```python
from build123d import *

# Parameters (mm, degrees)
EXTRUDE_1_DEPTH     = 10
EXTRUDE_2_DEPTH     = 13
EXTRUDE_3_DEPTH     = 9
EXTRUDE_4_DEPTH     = 9
SKETCH_7_R          = 74.5
SKETCH_7_R_2        = 62
EXTRUDE_5_DEPTH     = 16
SKETCH_8_R          = 62
CUT_EXTRUDE_1_DEPTH = 10
SKETCH_9_R          = 15
CUT_EXTRUDE_2_DEPTH = 10
SKETCH_10_R         = 2.5
CUT_EXTRUDE_3_DEPTH = 10
SKETCH_11_R         = 2.1
CUT_EXTRUDE_4_DEPTH = 10
SKETCH_12_R         = 2.5
CUT_EXTRUDE_5_DEPTH = 16
SKETCH_14_R         = 7
CUT_EXTRUDE_7_DEPTH = 13
SKETCH_16_R         = 5
CUT_EXTRUDE_9_DEPTH = 13


with BuildPart() as part:
    # ｽｹｯﾁ1 → ﾎﾞｽ - 押し出し1 (new body)
    with BuildSketch(Plane.XY):
        with BuildLine():
            Line((13, 0), (308, 0))
            Line((308, 0), (318, 10))
            Line((318, 10), (318, 348))
            Line((318, 348), (308, 358))
            Line((308, 358), (13, 358))
            Line((13, 358), (13, 214))
            Line((13, 214), (56, 214))
            ThreePointArc((56, 214), (63.071067812, 211.071067812), (66, 204))
            Line((66, 204), (66, 154))
            ThreePointArc((66, 154), (63.071067812, 146.928932188), (56, 144))
            Line((56, 144), (13, 144))
            Line((13, 144), (13, 0))
        make_face()
    extrude(amount=-EXTRUDE_1_DEPTH)

    # ｽｹｯﾁ2 → ﾎﾞｽ - 押し出し2 (add)
    with BuildSketch(Plane(origin=(0, 0, 0), x_dir=(0, 0, -1), z_dir=(1, 0, 0))):
        with BuildLine():
            Line((0, 0), (108, 0))
            ThreePointArc((108, 0), (115.071067812, 2.928932188), (118, 10))
            Line((118, 10), (118, 348))
            ThreePointArc((118, 348), (115.071067812, 355.071067812), (108, 358))
            Line((108, 358), (0, 358))
            Line((0, 358), (0, 0))
        make_face()
    extrude(amount=EXTRUDE_2_DEPTH)

    # ｽｹｯﾁ4 → ﾎﾞｽ - 押し出し3 (add)
    with BuildSketch(Plane(origin=(0, 40, 0), x_dir=(1, 0, 0), z_dir=(0, 1, 0))):
        Polygon((13, 10), (318, 10), (318, 108), (308, 118), (13, 118), align=None)
    extrude(amount=EXTRUDE_3_DEPTH)

    # ｽｹｯﾁ6 → ﾎﾞｽ - 押し出し4 (add)
    with BuildSketch(Plane(origin=(0, 309, 0), x_dir=(1, 0, 0), z_dir=(0, 1, 0))):
        Polygon((13, 10), (318, 10), (318, 108), (308, 118), (13, 118), align=None)
    extrude(amount=EXTRUDE_4_DEPTH)

    # ｽｹｯﾁ7 → ﾎﾞｽ - 押し出し5 (add)
    with BuildSketch(Plane.XY):
        with Locations((228, 179)):
            Circle(SKETCH_7_R)
        with Locations((228, 179)):
            Circle(SKETCH_7_R_2, mode=Mode.SUBTRACT)
    extrude(amount=-EXTRUDE_5_DEPTH)

    # ｽｹｯﾁ8 → ｶｯﾄ - 押し出し1 (cut)
    with BuildSketch(Plane.XY):
        with Locations((228, 179)):
            Circle(SKETCH_8_R)
    extrude(amount=-CUT_EXTRUDE_1_DEPTH, mode=Mode.SUBTRACT)

    # ｽｹｯﾁ9 → ｶｯﾄ - 押し出し2 (cut)
    with BuildSketch(Plane.XY):
        with Locations((122.891, 259.0915)):
            Circle(SKETCH_9_R)
    extrude(amount=-CUT_EXTRUDE_2_DEPTH, mode=Mode.SUBTRACT)

    # ｽｹｯﾁ10 → ｶｯﾄ - 押し出し3 (cut)
    with BuildSketch(Plane.XY):
        with Locations((103.6074, 236.1102)):
            Circle(SKETCH_10_R)
        with Locations((142.1746, 282.0728)):
            Circle(SKETCH_10_R)
    extrude(amount=-CUT_EXTRUDE_3_DEPTH, mode=Mode.SUBTRACT)

    # ｽｹｯﾁ11 → ｶｯﾄ - 押し出し4 (cut)
    with BuildSketch(Plane.XY):
        with Locations((108.5, 14.5)):
            Circle(SKETCH_11_R)
        with Locations((130, 35.5)):
            Circle(SKETCH_11_R)
    extrude(amount=-CUT_EXTRUDE_4_DEPTH, mode=Mode.SUBTRACT)

    # ｽｹｯﾁ12 → ｶｯﾄ - 押し出し5 (cut)
    with BuildSketch(Plane.XY):
        with Locations((295.5, 179)):
            Circle(SKETCH_12_R)
        with Locations((275.7297, 226.7297)):
            Circle(SKETCH_12_R)
        with Locations((228, 246.5)):
            Circle(SKETCH_12_R)
        with Locations((180.2703, 226.7297)):
            Circle(SKETCH_12_R)
        with Locations((160.5, 179)):
            Circle(SKETCH_12_R)
        with Locations((180.2703, 131.2703)):
            Circle(SKETCH_12_R)
        with Locations((228, 111.5)):
            Circle(SKETCH_12_R)
        with Locations((275.7297, 131.2703)):
            Circle(SKETCH_12_R)
    extrude(amount=-CUT_EXTRUDE_5_DEPTH, mode=Mode.SUBTRACT)

    # ｽｹｯﾁ14 → ｶｯﾄ - 押し出し7 (cut)
    with BuildSketch(Plane(origin=(0, 0, 0), x_dir=(0, 0, -1), z_dir=(1, 0, 0))):
        with Locations((30, 15)):
            Circle(SKETCH_14_R)
        with Locations((100, 15)):
            Circle(SKETCH_14_R)
        with Locations((30, 343)):
            Circle(SKETCH_14_R)
        with Locations((100, 343)):
            Circle(SKETCH_14_R)
        with Locations((100, 123)):
            Circle(SKETCH_14_R)
        with Locations((100, 235)):
            Circle(SKETCH_14_R)
    extrude(amount=CUT_EXTRUDE_7_DEPTH, mode=Mode.SUBTRACT)

    # ｽｹｯﾁ16 → ｶｯﾄ - 押し出し9 (cut)
    with BuildSketch(Plane(origin=(0, 0, 0), x_dir=(0, 0, -1), z_dir=(1, 0, 0))):
        with Locations((65, 15)):
            Circle(SKETCH_16_R)
        with Locations((65, 343)):
            Circle(SKETCH_16_R)
    extrude(amount=CUT_EXTRUDE_9_DEPTH, mode=Mode.SUBTRACT)


solid = part.part
```
Design review of the part built by this model. Coordinates are the model's own, in mm. A direction names the side the tool comes from. Round coordinates to 2 decimals unless told otherwise and drop trailing zeros. Write each loop counter-clockwise with the first axis right and the second up, starting at its lowest first coordinate (ties: lowest second). Pieces come first, ordered by that corner, then holes. Notation, with made-up numbers: (74, -9) -> (91, -9) arc R11 cw to (91, 7) -> close; hole circle Ø6 at (54.25, -1). An arc over 180 degrees is marked (long way). Answer in a Markdown table with one row per item.
Q1. Draft analysis for pull direction Y (two halves, no side actions). For faces 4 (the face through (163, 40, -65)), 5 (the face through (163, 318, -65)), 6 (the face through (163, 20, -10)), 7 (the face through (6.41, 10.12, -63.92)), state which applies: +Y half, -Y half, draft (parallel to the pull), parting line (faces both ways), or undercut.
The answers:
| item | result |
|---|---|
| face 4 | -Y half |
| face 5 | +Y half |
| face 6 | draft |
| face 7 | undercut |
Q2. Take a section at B-B, the plane y = 269.5. State the section outline as (x, z) points, then the cut area to 3 significant figures.
The answers:
| item | result |
|---|---|
| outline | (0, -118) -> (13, -118) -> (13, -10) -> (112.09, -10) -> (112.09, 0) -> (0, 0) -> close; (133.69, -10) -> (318, -10) -> (318, 0) -> (133.69, 0) -> close |
| area | 4,370 mm² |
Q3. Take a section at C-C, the plane x = 212. State the section outline as (y, z) points, then the cut area to 3 significant figures.
The answers:
| item | result |
|---|---|
| outline | (0, -10) -> (40, -10) -> (40, -118) -> (49, -118) -> (49, -10) -> (106.24, -10) -> (106.24, -16) -> (119.1, -16) -> (119.1, 0) -> (0, 0) -> close; (238.9, -16) -> (251.76, -16) -> (251.76, -10) -> (309, -10) -> (309, -118) -> (318, -118) -> (318, -10) -> (358, -10) -> (358, 0) -> (238.9, 0) -> close |
| area | 4,480 mm² |
Q4. For faces 1 (the face through (184, 223, -16)), 2 (the face through (129, 181, -10)), 3 (the face through (66, 179, -5)), list the 3-axis set-ups (+Z, -Z, +X, -X, +Y, -Y) from which the entire face can be reached by the end or side of a thin tool; tool diameter is ignored.
The answers:
| item | result |
|---|---|
| face 1 | -Z, +X |
| face 2 | -Z |
| face 3 | +Z, -Z |
Q5. Clearance check with flat-ended pins moving along their axes: pin 1 Ø1 at (x, y) = (94.5, 119) entering from -Z; pin 2 Ø3 at (x, y) = (275.73, 226.73) entering from -Z; pin 3 Ø16 at (y, z) = (343, -100) entering from +X; pin 4 Ø6.5 at (x, y) = (275.73, 131.27) entering from -Z. State where each tip first meets the part, or that it passes through.
The answers:
| item | result |
|---|---|
| pin 1 | z = -10 |
| pin 2 | through |
| pin 3 | x = 13 |
| pin 4 | z = -16 |
Q6. Take a section at D-D, the plane z = -65. State the section outline as (x, y) points.
The answers:
| item | result |
|---|---|
| outline | (0, 0) -> (13, 0) -> (13, 10) -> (0, 10) -> close; (0, 20) -> (13, 20) -> (13, 40) -> (318, 40) -> (318, 49) -> (13, 49) -> (13, 309) -> (318, 309) -> (318, 318) -> (13, 318) -> (13, 338) -> (0, 338) -> close; (0, 348) -> (13, 348) -> (13, 358) -> (0, 358) -> close |
Q7. To check wall thickness, follow L1, parallel to Y at x = 8, z = -100; L2, parallel to Z at x = 8, y = 343; L3, parallel to Y at x = 146, z = -16. State the ranges of each line that lie inside material, in increasing order. Write a range as [from, to].
The answers:
| item | result |
|---|---|
| L1 | [0, 8], [22, 116], [130, 228], [242, 336], [350, 358] |
| L2 | [-118, -107], [-93, -70], [-60, -37], [-23, 0] |
| L3 | [40, 49], [309, 318] |
Q8. Take a section at A-A, the plane z = -30. State the section outline as (x, y) points, then the cut area to 3 significant figures.
The answers:
| item | result |
|---|---|
| outline | (0, 0) -> (13, 0) -> (13, 8) -> (0, 8) -> close; (0, 22) -> (13, 22) -> (13, 40) -> (318, 40) -> (318, 49) -> (13, 49) -> (13, 309) -> (318, 309) -> (318, 318) -> (13, 318) -> (13, 336) -> (0, 336) -> close; (0, 350) -> (13, 350) -> (13, 358) -> (0, 358) -> close |
| area | 9,780 mm² |
